Geometry check sheet. Reference: drawing and pictorial views, mm from the part's lowest x, y, z. A direction names the side the tool comes from. Give positions to 0.01 mm unless a question says otherwise; leave off trailing zeros. Write each loop counter-clockwise with the first axis right and the second up, starting at its lowest first coordinate (ties: lowest second). Pieces come first, ordered by that corner, then holes. Notation, with made-up numbers: M -4,43.25 L 28,43.25 A28 ccw 28,73.25 Z; hole C 55,87.25 d9. An arc over 180 degrees is marked long. Answer as a JSON object with one key per item and string values.
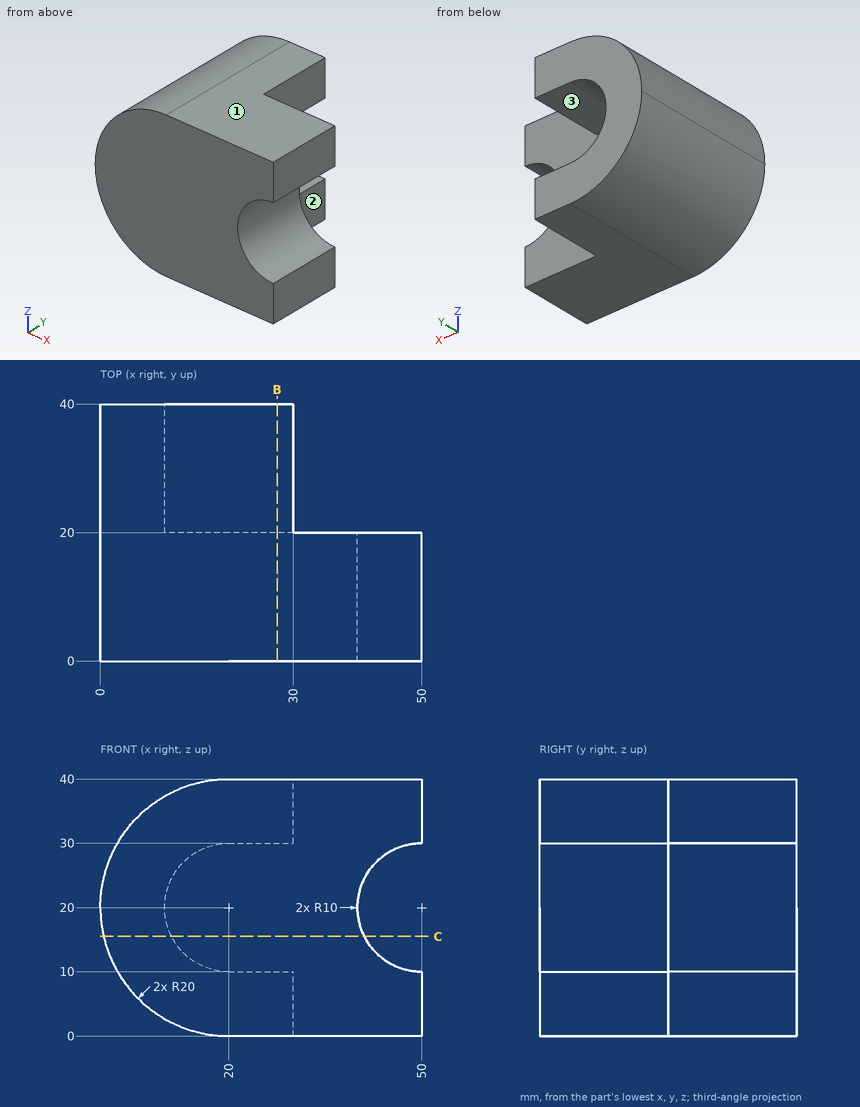
1) Thickness scan on L1, parallel to Y at x = 34, z = 31; L2, parallel to Z at x = 43.5, y = 14.5; L3, parallel to Z at x = 23.5, y = 21.5. Record the ranges inside material, lowest first.
Completed:
{"L1": "y = 0 to 20", "L2": "z = 0 to 12.4, 27.6 to 40", "L3": "z = 0 to 10, 30 to 40"}
2) Go/stop test with flat-tipped pins: pin 1 (1.5 mm diameter, centred on y = 31, z = 34.5, fed in from +X); pin 2 (1.5 mm diameter, centred on x = 12.5, y = 6.5, fed in from -Z); pin 3 (10 mm diameter, centred on x = 41, z = 19.5, fed in from +Y). Record where each tip stops, or that it passes through.
Completed:
{"pin 1": "stops at x = 30", "pin 2": "stops at z = 1.17", "pin 3": "stops at y = 20"}
3) Section check B-B on x = 27.5. Record the boundary of the cut face in (y, z).
Completed:
{"outline": "M 0,0 L 40,0 L 40,10 L 20,10 L 20,30 L 40,30 L 40,40 L 0,40 Z"}
4) Access from +Z, -Z, +X, -X, +Y, -Y to the whole of each face (thin tool, end or side, straight path). Record for the marked faces 1, 2 and 3.
Completed:
{"face 1": "+Z, +X, -X, +Y, -Y", "face 2": "+Z, -Z, +X, +Y", "face 3": "+X, +Y"}
5) Section check C-C on z = 15.5. Record the boundary of the cut face in (x, y).
Completed:
{"outline": "M 0.51,0 L 41.07,0 L 41.07,20 L 11.07,20 L 11.07,40 L 0.51,40 Z"}
